```python
from build123d import *

# Parameters (mm, degrees)
SKETCH2_W           = 59.5
SKETCH2_H           = 39.5
BOSS_EXTRUDE1_DEPTH = 3
FILLET1_R           = 3
CHAMFER1_SIZE       = 0.5
SKETCH3_W           = 14
SKETCH3_H           = 17.5
SKETCH3_W_2         = 15
BOSS_EXTRUDE2_DEPTH = 10.5
CUT_EXTRUDE1_REACH  = 43.077
SKETCH4_W           = 14
SKETCH4_H           = 3.577165811
SKETCH4_W_2         = 14.5
SKETCH4_H_2         = 14.5
SKETCH5_W           = 12
SKETCH5_H           = 15
CUT_EXTRUDE2_DEPTH  = 1.5
SKETCH6_W           = 7
SKETCH6_H           = 17.5
CUT_EXTRUDE3_DEPTH  = 10
SKETCH7_W           = 7
SKETCH7_H           = 17.5
CUT_EXTRUDE4_DEPTH  = 10


with BuildPart() as part:
    # Sketch2 → Boss-Extrude1 (new body)
    with BuildSketch(Plane.XY.offset(122.238514037)):
        with Locations((-4.628679656, 0.128679656)):
            Rectangle(SKETCH2_W, SKETCH2_H)
    extrude(amount=BOSS_EXTRUDE1_DEPTH)

    # Fillet1
    fillet1_edges = [part.edges().sort_by_distance(p)[0] for p in [
        (-34.378679656, 19.878679656, 123.738514037),
        (25.121320344, 19.878679656, 123.738514037),
        (25.121320344, -19.621320344, 123.738514037),
        (-34.378679656, -19.621320344, 123.738514037),
    ]]
    fillet(fillet1_edges, radius=FILLET1_R)

    # Chamfer1
    chamfer1_edges = [part.edges().sort_by_distance(p)[0] for p in [
        (-34.378679656, 0.128679656, 122.238514037),
        (-4.628679656, 19.878679656, 122.238514037),
        (25.121320344, 0.128679656, 122.238514037),
        (-4.628679656, -19.621320344, 122.238514037),
        (-33.5, -18.742640687, 122.238514037),
        (24.242640687, -18.742640687, 122.238514037),
        (24.242640687, 19, 122.238514037),
        (-33.5, 19, 122.238514037),
    ]]
    chamfer(chamfer1_edges, length=CHAMFER1_SIZE)

    # Sketch3 → Boss-Extrude2 (add)
    with BuildSketch(Plane(origin=(0, 0, 122.238514037), x_dir=(-1, 0, 0), z_dir=(0, 0, -1))):
        with Locations((-16.621320344, 5.628679656)):
            Rectangle(SKETCH3_W, SKETCH3_H)
        with Locations((25.378679656, 5.628679656)):
            Rectangle(SKETCH3_W_2, SKETCH3_H)
    extrude(amount=BOSS_EXTRUDE2_DEPTH)

    # Sketch4 → Cut-Extrude1 (cut, up to next)
    with BuildSketch(Plane(origin=(0, 0, 122.238514037), x_dir=(-1, 0, 0), z_dir=(0, 0, -1)), mode=Mode.PRIVATE) as cut_extrude1_sk1:
        with Locations((4.628679656, -17.832737439)):
            Rectangle(SKETCH4_W, SKETCH4_H)
    cut_extrude1_tool1 = extrude(cut_extrude1_sk1.sketch, amount=-CUT_EXTRUDE1_REACH, mode=Mode.PRIVATE) & part.part
    # Sketch4 → Cut-Extrude1 (cut, up to next)
    with BuildSketch(Plane(origin=(0, 0, 122.238514037), x_dir=(-1, 0, 0), z_dir=(0, 0, -1)), mode=Mode.PRIVATE) as cut_extrude1_sk2:
        with Locations((4.628679656, 2.628679656)):
            Rectangle(SKETCH4_W_2, SKETCH4_H_2)
    cut_extrude1_tool2 = extrude(cut_extrude1_sk2.sketch, amount=-CUT_EXTRUDE1_REACH, mode=Mode.PRIVATE) & part.part
    add(cut_extrude1_tool1.solids().sort_by_distance((-4.62868, -17.832737, 122.238514))[0], mode=Mode.SUBTRACT)
    add(cut_extrude1_tool2.solids().sort_by_distance((-4.62868, 2.62868, 122.238514))[0], mode=Mode.SUBTRACT)

    # Sketch5 → Cut-Extrude2 (cut)
    with BuildSketch(Plane(origin=(0, 0, 122.238514037), x_dir=(-1, 0, 0), z_dir=(0, 0, -1))):
        with Locations((4.628679656, -8.544154533)):
            Rectangle(SKETCH5_W, SKETCH5_H)
    extrude(amount=-CUT_EXTRUDE2_DEPTH, mode=Mode.SUBTRACT)

    # Sketch6 → Cut-Extrude3 (cut)
    with BuildSketch(Plane.ZY.offset(-9.621320344)):
        with Locations((117.238514037, 5.628679656)):
            Rectangle(SKETCH6_W, SKETCH6_H)
    extrude(amount=-CUT_EXTRUDE3_DEPTH, mode=Mode.SUBTRACT)

    # Sketch7 → Cut-Extrude4 (cut)
    with BuildSketch(Plane(origin=(-17.878679656, 0, 0), x_dir=(0, 0, -1), z_dir=(1, 0, 0))):
        with Locations((-117.238514037, 5.628679656)):
            Rectangle(SKETCH7_W, SKETCH7_H)
    extrude(amount=-CUT_EXTRUDE4_DEPTH, mode=Mode.SUBTRACT)


solid = part.part
```
Design review of the part built by this model. Coordinates are the model's own, in mm. A direction names the side the tool comes from. Coordinates: 2 decimals unless noted, no trailing zeros. Write each loop counter-clockwise with the first axis right and the second up, starting at its lowest first coordinate (ties: lowest second). Pieces come first, ordered by that corner, then holes.
1) Add section C-C (y = 12.5). Write out the cut boundary in (x, z).
2) Add section B-B (x = 16.5). Write out the cut boundary in (y, z), plus the area to 4 significant figures.
3) Add section A-A (z = 119.5). Write out the cut boundary in (x, y), plus the area to 4 significant figures.
4) Mouldability with a two-part tool opening along X and no side actions: class faces 5 (the conical face through (-33.26, 18.72, 122.37)), 6 (the flat face through (-17.879, 6, 121)), 7 (the flat face through (-29, -3.121, 117)), 8 (the flat face through (-11.879, 3, 124)) as +X half, -X half, draft (parallel to the pull), parting line (faces both ways), or undercut.
5) Insertion check: pin 1 (0.9 mm diameter, centred on x = -7, z = 123.5, fed in from -Y); pin 2 (5 mm diameter, centred on x = 17.5, z = 117.5, fed in from +Y); pin 3 (1.2 mm diameter, centred on y = 10, z = 121.5, fed in from +X); pin 4 (12 mm diameter, centred on x = 6.5, y = -5, fed in from -Z). Each pin has a flat end and moves straight along its axis. Give the tip position at first contact, or say it passes through.
6) Machinability: for faces 1 (the flat face through (15, 6, 113.739)), 2 (the flat face through (-5, -16.044, 124)), 3 (the flat face through (-32.879, 6, 117)), 4 (the flat face through (23.621, 6, 117)), which of the approach directions +Z, -Z, +X, -X, +Y, -Y give a long, thin tool a straight path to every point of the face, cutting with its end or side? Answer none if there is none.
7) To check wall thickness, follow L1, parallel to Z at x = 10, y = 8.5; L2, parallel to X at y = 4.5, z = 120.25; L3, parallel to Z at x = -6.5, y = 18. State the ranges of each line that lie inside material, in increasing order.
8) Add section D-D (x = 7). Write out the cut boundary in (y, z).
Check result:
1. outline: (-34.38, 122.74) - (-33.88, 122.24) - (-32.88, 122.24) - (-32.88, 111.74) - (-17.88, 111.74) - (-17.88, 113.74) - (-27.88, 113.74) - (-27.88, 120.74) - (-17.88, 120.74) - (-17.88, 122.24) - (9.62, 122.24) - (9.62, 120.74) - (19.62, 120.74) - (19.62, 113.74) - (9.62, 113.74) - (9.62, 111.74) - (23.62, 111.74) - (23.62, 122.24) - (24.62, 122.24) - (25.12, 122.74) - (25.12, 125.24) - (-34.38, 125.24) - close
2. outline: (-19.62, 122.74) - (-19.12, 122.24) - (-3.12, 122.24) - (-3.12, 120.74) - (14.38, 120.74) - (14.38, 122.24) - (19.38, 122.24) - (19.88, 122.74) - (19.88, 125.24) - (-19.62, 125.24) - close; (-3.12, 111.74) - (14.38, 111.74) - (14.38, 113.74) - (-3.12, 113.74) - close
2. area: 179.5 mm2
3. outline: (-32.88, -3.12) - (-27.88, -3.12) - (-27.88, 14.38) - (-32.88, 14.38) - close; (19.62, -3.12) - (23.62, -3.12) - (23.62, 14.38) - (19.62, 14.38) - close
3. area: 157.5 mm2
4. face 5: -X half
4. face 6: undercut
4. face 7: draft
4. face 8: undercut
5. pin 1: stops at y = -16.04
5. pin 2: stops at y = 14.38
5. pin 3: stops at x = 23.62
5. pin 4: stops at z = 111.74
6. face 1: +Y, -Y
6. face 2: +Z, -Z, -Y
6. face 3: -Z, -X, +Y, -Y
6. face 4: -Z, +X, +Y, -Y
7. L1: z = 111.74 to 113.74, 120.74 to 125.24
7. L2: x = -32.88 to -27.88, 19.62 to 23.62
7. L3: z = 122.24 to 125.24
8. outline: (-19.62, 122.74) - (-19.12, 122.24) - (19.38, 122.24) - (19.88, 122.74) - (19.88, 125.24) - (-19.62, 125.24) - close
